Verification items for the finished model (mm, model axes). A direction names the side the tool comes from. Round coordinates to 2 decimals unless told otherwise and drop trailing zeros. Order: outer loops, then holes, each group sorted by start corner. A loop starts at its lowest first (then second) coordinate and runs counter-clockwise, first axis right, second up. Notation, with made-up numbers: (-21, 47.25) -> (-11, 47.25) arc R24 cw to (-11, 85.25) -> close; hole circle Ø8 at (52.25, -11). An arc over 180 degrees is marked (long way). Return JSON: item names as keys, results as strings. Group by question number.
Item 1: Sectioned sample at C-C on x = -5.5. Record the cut outline in (y, z).
Item 2: Sectioned sample at D-D on y = -12. Record the cut outline in (x, z).
Item 3: Draft check along X on faces 1 (the flat face through (0, -15.022, -10)), 2 (the cylindrical face through (0.36, 1.68, -10.19)). Enter one of: pulls with the +X half, pulls with the -X half, needs draft (parallel to the pull), parting line crosses it, or undercut.
Item 4: Sectioned sample at A-A on y = -1. Record the cut outline in (x, z).
Item 5: Depth check by flat-ended pin: pin 1 Ø5 at (x, y) = (-2, 0.5) entering from +Z; pin 2 Ø2 at (x, y) = (-4.5, -9.5) entering from -Z. Enter the tip coordinate at first touch or a pass-through.
Item 6: Sectioned sample at B-B on y = -5.5. Record the cut outline in (x, z), plus the area to 3 significant figures.
Item 7: Scan lines: probe 1 along X at (y, z) = (-11, -8.55); probe 2 along Z at (x, y) = (1.5, 3.5); probe 3 along Y at (x, z) = (0.5, -10.15). Record each from-to range of solid material in increasing order. Write a range as from..to.
Item 8: Access from +Z, -Z, +X, -X, +Y, -Y to the whole of each face (thin tool, end or side, straight path). Record for faces 3 (the flat face through (0, 15.022, -10)), 4 (the flat face through (0, -5.222, -9)).
Autodesk Inventor part; units mm, degrees
ref_plane "YZ Plane" through (0, 0, 0) normal (1, 0, 0) x (0, 1, 0)
ref_plane "XZ Plane" through (0, 0, 0) normal (0, 1, 0) x (-1, 0, 0)
ref_plane "XY Plane" through (0, 0, 0) normal (0, 0, 1) x (1, 0, 0)
ref_plane "Work Plane2" through (-0.0047, 0, -9.2) normal (-0.001, 0, -1) x (-1, 0, 0.001)
sketch "Sketch2" plane through (-0.0047, 0, -9.2) normal (-0.001, 0, -1) x (-1, 0, 0.001)
  line L0 (6, 2.0218) -> (3.5, 15.0218)
  line L1 (6, -1.9782) -> (6, 2.0218)
  line L2 (2.5, -15.0218) -> (6, -1.9782)
  line L3 (3.5, 15.0218) -> (-3.5, 15.0218)
  line L4 (-3.5, 15.0218) -> (-6, 2.0218)
  line L5 (-6, 2.0218) -> (-6, -1.9782)
  line L6 (-6, -1.9782) -> (-2.5, -15.0218)
  line L7 (1.25, -15.0218) -> (2.5, -15.0218)
  line L8 (-2.5, -15.0218) -> (-1.25, -15.0218)
  line L9 (1.25, -15.0218) -> (-1.25, -15.0218)
  circle A0 centre (0, 0.0218) radius 1.7
  point P0 (0.0047, 0)
extrude "Extrusion1" add sketch "Sketch2" along normal blind 2
sketch "Sketch3" plane through (-0.0047, 0, -9.2) normal (0.001, 0, 1) x (1, 0, -0.001)
  line L0 (1.25, -15.0218) -> (1.25, -5.0218) construction
  line L1 (-1.25, -5.0218) -> (-1.25, -15.0218) construction
  line L2 (2.5, -15.0218) -> (-2.5, -15.0218)
  line L3 (1.05, -5.2218) -> (-1.05, -5.2218)
  line L4 (-1.05, -5.2218) -> (-1.05, -15.0218)
  line L5 (-1.05, -15.0218) -> (1.05, -15.0218)
  line L6 (1.05, -15.0218) -> (1.05, -5.2218)
  point P0 (-0.0047, 0)
  point P1 (1.05, -15.0218)
  dimension "d2" = 0.2
  dimension "d3" = 0.2
  dimension "d4" = 0.2
extrude "Extrusion2" add sketch "Sketch3" along normal blind 1
equation "\"d3\" = d2"
equation "\"d4\" = d2"
properties part number "SmallBeltClampCover"
Recorded:
{
 "1": {"outline": "(-3.87, -11.19) -> (4.66, -11.19) -> (4.65, -9.19) -> (-3.86, -9.19) -> close"},
 "2": {"outline": "(-3.32, -11.2) -> (3.3, -11.2) -> (3.31, -9.2) -> (1.05, -9.2) -> (1.05, -8.2) -> (-1.05, -8.2) -> (-1.05, -9.2) -> (-3.32, -9.2) -> close"},
 "3": {"face 1": "needs draft", "face 2": "undercut"},
 "4": {"outline": "(-6.01, -11.19) -> (-1.37, -11.2) -> (-1.36, -9.2) -> (-6, -9.19) -> close; (1.35, -11.2) -> (5.99, -11.21) -> (6, -9.21) -> (1.35, -9.2) -> close"},
 "5": {"pin 1": "z = -9.2", "pin 2": "z = -11.2"},
 "6": {"outline": "(-5.06, -11.19) -> (5.05, -11.21) -> (5.05, -9.21) -> (1.05, -9.2) -> (1.05, -8.2) -> (-1.05, -8.2) -> (-1.05, -9.2) -> (-5.06, -9.19) -> close", "area": "22.3 mm²"},
 "7": {"probe 1": "-1.05..1.05", "probe 2": "-11.2..-9.2", "probe 3": "-15.02..-1.6, 1.64..15.02"},
 "8": {"face 3": "+Z, -Z, +X, -X, +Y", "face 4": "+Z, +X, -X, +Y"}
}
